The listing builds one solid part. Answer for the finished solid, in the listing's coordinates (mm). A direction names the side the tool comes from. Give positions to 0.01 mm unless a question says otherwise; leave off trailing zeros. Write each loop counter-clockwise with the first axis right and the second up, starting at its lowest first coordinate (ties: lowest second). Pieces come first, ordered by that corner, then holes. Notation, with made-up numbers: (-39.5, 67.25) -> (-30.5, 67.25) arc R23 ccw to (-30.5, 86.25) -> close; hole circle Ø7 at (32, 11.5). An arc over 180 degrees is marked (long way). Put each result on its own line as item: value. Start each with the question number.
1) For a pull along X with two mould halves and no side action, classify faces 6 (the flat face through (31.75, 3, -12)), 7 (the cylindrical face through (-91.987, 3.131, -80.347)), 8 (the flat face through (113, 3, -78.232)) as released by +X, released by -X, zero draft, split by the parting line, or undercut.
2) For faces 1 (the flat face through (-11, 6.35, -17)), 2 (the flat face through (-6, 3, -19.05)), 3 (the flat face through (109.775, 3, -73)), 4 (the flat face through (109.775, 3, -96)), 5 (the flat face through (-11, 0, -17)), determine the directions among +Z, -Z, +X, -X, +Y, -Y from which every point of the face is accessible in a straight line to the end or side of a thin tool.
3) Flat-ended cylindrical pins translate along their axes: pin 1 Ø3 at (y, z) = (4, -10.5) entering from -X; pin 2 Ø2 at (x, y) = (57.5, 3.5) entering from +Z; pin 3 Ø3 at (x, y) = (27.5, 4.5) entering from -Z. Find the tip coordinate at first contact, or state that the pin passes through.
4) A cutting plane is placed at B-B (x = 89.5). Write down the section's boundary in (y, z).
5) A cutting plane is placed at A-A (z = -13.5). Write down the section's boundary in (x, y), then the cut area to 3 significant figures.
6) A cutting plane is placed at D-D (y = 2). Write down the section's boundary in (x, z) (3 decimals), then the cut area to 3 significant figures.
7) Find the intervals of material crossed by line 1 along X through (y, z) = (2.5, -85.5); line 2 along X through (y, z) = (0.5, -16); line 3 along X through (y, z) = (0.75, -97), in increasing order. Write a range as from..to.
8) A cutting plane is placed at C-C (z = -140). Write down the section's boundary in (x, y), then the cut area to 3 significant figures.
from build123d import *

# Parameters (mm, degrees)
BOSS_EXTRUDE1_DEPTH = 6.35


with BuildPart() as part:
    # Sketch1 → Boss-Extrude1 (new body)
    with BuildSketch(Plane(origin=(0, 0, 0), x_dir=(1, 0, 0), z_dir=(0, 1, 0))):
        with BuildLine():
            Line((109.774588029, 101.091898562), (109.774588029, 90.931898562))
            Line((109.774588029, 90.931898562), (116.124588029, 90.931898562))
            Line((116.124588029, 90.931898562), (116.124588029, 78.231898562))
            Line((116.124588029, 78.231898562), (109.774588029, 78.231898562))
            Line((109.774588029, 78.231898562), (109.774588029, 68.071898562))
            ThreePointArc((109.774588029, 68.071898562), (-92.075, 84.581898562), (109.774588029, 101.091898562))
        make_face()
        with BuildLine():
            Line((0, 0), (19.05, 0))
            Line((19.05, 0), (19.05, 19.05))
            Line((19.05, 19.05), (31.75, 19.05))
            Line((31.75, 19.05), (31.75, 5.08))
            ThreePointArc((31.75, 5.08), (9.525, 167.131898562), (-12.7, 5.08))
            Line((-12.7, 5.08), (-12.7, 19.05))
            Line((-12.7, 19.05), (0, 19.05))
            Line((0, 19.05), (0, 0))
        make_face(mode=Mode.SUBTRACT)
    extrude(amount=BOSS_EXTRUDE1_DEPTH)


solid = part.part
Reply:
1. face 6: undercut
1. face 7: split by the parting line
1. face 8: zero draft
2. face 1: +Z, -Z, +X, -X, +Y
2. face 2: +Y, -Y
2. face 3: +Z, +X, +Y, -Y
2. face 4: -Z, +X, +Y, -Y
2. face 5: +Z, -Z, +X, -X, -Y
3. pin 1: stops at x = -61.57
3. pin 2: stops at z = 5.51
3. pin 3: stops at z = -184.84
4. outline: (0, -147.24) -> (6.35, -147.24) -> (6.35, -105.04) -> (0, -105.04) -> close; (0, -64.12) -> (6.35, -64.12) -> (6.35, -21.92) -> (0, -21.92) -> close
5. outline: (-63.07, 0) -> (-32.45, 0) -> (-32.45, 6.35) -> (-63.07, 6.35) -> close; (-12.7, 0) -> (0, 0) -> (0, 6.35) -> (-12.7, 6.35) -> close; (19.05, 0) -> (31.75, 0) -> (31.75, 6.35) -> (19.05, 6.35) -> close; (51.5, 0) -> (82.12, 0) -> (82.12, 6.35) -> (51.5, 6.35) -> close
5. area: 550 mm2
6. outline: (109.775, -101.092) -> (109.775, -90.932) -> (116.125, -90.932) -> (116.125, -78.232) -> (109.775, -78.232) -> (109.775, -68.072) arc R101.6 ccw (long way) to start; hole (-12.7, -19.05) -> (-12.7, -5.08) arc R82.55 ccw (long way) to (31.75, -5.08) -> (31.75, -19.05) -> (19.05, -19.05) -> (19.05, 0) -> (0, 0) -> (0, -19.05) -> close
6. area: 11,400 mm2
7. line 1: x = -92.07..-73.02, 92.07..116.12
7. line 2: x = -65.44..-36.42, -12.7..0, 19.05..31.75, 55.47..84.49
7. line 3: x = -91.31..-72.09, 91.14..109.77
8. outline: (-75.63, 0) -> (-51.66, 0) -> (-51.66, 6.35) -> (-75.63, 6.35) -> close; (70.71, 0) -> (94.68, 0) -> (94.68, 6.35) -> (70.71, 6.35) -> close
8. area: 304 mm2
